Autodesk Fusion 360 part; units mm, degrees
sketch "Sketch1" plane through (0, 0, 0) normal (0, 0, 1) x (1, 0, 0)
  line L0 (-0.5032, -3.4999) -> (2.3969, -3.5062) construction
  line L1 (3.8936, -5.0095) -> (3.8707, -15.5094) construction
  line L2 (5.3674, -17.0127) -> (32.3673, -17.0717) construction
  line L3 (33.8706, -15.575) -> (33.8935, -5.075) construction
  line L4 (35.3968, -3.5783) -> (37.3968, -3.5826) construction
  line L5 (38.8935, -5.0859) -> (38.8706, -15.5859) construction
  line L6 (40.3673, -17.0892) -> (58.8673, -17.1296) construction
  arc A0 (3.8707, -15.5094) -> (5.3674, -17.0127) centre (5.3707, -15.5127) ccw construction
  arc A1 (3.8936, -5.0095) -> (2.3969, -3.5062) centre (2.3936, -5.0062) ccw construction
  arc A2 (32.3673, -17.0717) -> (33.8706, -15.575) centre (32.3706, -15.5717) ccw construction
  arc A3 (35.3968, -3.5783) -> (33.8935, -5.075) centre (35.3935, -5.0783) ccw construction
  arc A4 (38.8935, -5.0859) -> (37.3968, -3.5826) centre (37.3935, -5.0826) ccw construction
  arc A5 (38.8706, -15.5859) -> (40.3673, -17.0892) centre (40.3706, -15.5892) ccw construction
  arc A6 (4.6436, -5.0111) -> (2.3985, -2.7562) centre (2.3936, -5.0062) ccw
  line L7 (-0.5049, -4.2499) -> (2.3952, -4.2562)
  line L8 (-0.5016, -2.7499) -> (2.3985, -2.7562)
  arc A7 (3.1436, -5.0078) -> (2.3952, -4.2562) centre (2.3936, -5.0062) ccw
  line L9 (3.1436, -5.0078) -> (3.1207, -15.5078)
  arc A8 (3.1207, -15.5078) -> (5.3658, -17.7627) centre (5.3707, -15.5127) ccw
  line L10 (5.3658, -17.7627) -> (32.3657, -17.8217)
  line L11 (4.6436, -5.0111) -> (4.6207, -15.5111)
  arc A9 (4.6207, -15.5111) -> (5.369, -16.2627) centre (5.3707, -15.5127) ccw
  line L12 (5.369, -16.2627) -> (32.369, -16.3217)
  arc A10 (32.369, -16.3217) -> (33.1206, -15.5733) centre (32.3706, -15.5717) ccw
  line L13 (33.1206, -15.5733) -> (33.1435, -5.0734)
  arc A11 (35.3984, -2.8283) -> (33.1435, -5.0734) centre (35.3935, -5.0783) ccw
  line L14 (35.3984, -2.8283) -> (37.3984, -2.8326)
  arc A12 (39.6435, -5.0876) -> (37.3984, -2.8326) centre (37.3935, -5.0826) ccw
  line L15 (39.6435, -5.0876) -> (39.6206, -15.5875)
  arc A13 (39.6206, -15.5875) -> (40.3689, -16.3392) centre (40.3706, -15.5892) ccw
  line L16 (40.3689, -16.3392) -> (58.8689, -16.3796)
  arc A14 (32.3657, -17.8217) -> (34.6206, -15.5766) centre (32.3706, -15.5717) ccw
  line L17 (34.6206, -15.5766) -> (34.6435, -5.0766)
  arc A15 (35.3952, -4.3283) -> (34.6435, -5.0766) centre (35.3935, -5.0783) ccw
  line L18 (35.3952, -4.3283) -> (37.3952, -4.3326)
  arc A16 (38.1435, -5.0843) -> (37.3952, -4.3326) centre (37.3935, -5.0826) ccw
  line L19 (38.1435, -5.0843) -> (38.1206, -15.5843)
  arc A17 (38.1206, -15.5843) -> (40.3657, -17.8392) centre (40.3706, -15.5892) ccw
  line L20 (40.3657, -17.8392) -> (58.8656, -17.8796)
  line L21 (58.8689, -16.3796) -> (58.8656, -17.8796)
  line L22 (-0.5016, -2.7499) -> (-0.4994, -1.7499) construction
  line L23 (-0.5049, -4.2499) -> (-0.4939, 0.7501) construction
  arc A18 (-0.4972, -0.7499) -> (-0.5016, -2.7499) centre (-0.4994, -1.7499) ccw
  arc A19 (-0.4939, 0.7501) -> (-0.5049, -4.2499) centre (-0.4994, -1.7499) ccw
  line L24 (-0.4972, -0.7499) -> (1.5028, -0.7542)
  line L25 (-0.4939, 0.7501) -> (1.5061, 0.7458)
  arc A20 (1.5028, -0.7542) -> (1.5061, 0.7458) centre (1.5044, -0.0042) ccw
  point P0 (3.8969, -3.5095)
  point P1 (3.8674, -17.0094)
  point P2 (33.8673, -17.075)
  point P3 (33.8968, -3.575)
  point P4 (38.8968, -3.5859)
  point P5 (38.8673, -17.0859)
  dimension "d34" = 30
  dimension "d35" = 13.5
  dimension "d36" = 5
  dimension "d37" = 13.5
  dimension "d38" = 20
  dimension "d39" = 1.5
  dimension "d40" = 1.5
  dimension "d41" = 1.5
  dimension "d42" = 1.5
  dimension "d43" = 1.5
  dimension "d44" = 1.5
  dimension "d49" = 0.75
  dimension "d52" = 0.75
  dimension "d53" = -0.75
  dimension "d54" = -0.75
  dimension "d55" = 0.75
  dimension "d56" = -0.75
  dimension "d57" = 0.75
  dimension "d58" = 0.75
  dimension "d59" = 1
  dimension "d60" = 2
  dimension "d62" = 5
  dimension "d67" = 2
  dimension "d68" = 2
extrude "Extrude1" add sketch "Sketch1" along normal blind 20
mirror "Mirror1" about plane through (58.8689, -16.3796, 0) normal (1, -0.0022, 0) of bodies 1 merged
equation "i1 = 2 mm"
equation "i2 = 5 mm"
equation "i3 = 30 mm"
equation "d34 = i3"
equation "d35 = h - t"
equation "d36 = i2"
equation "d37 = h - t"
equation "d38 = i / 2 - 2 * i2 - i3"
equation "d39 = Radial Dimension-2"
equation "d40 = Radial Dimension-3"
equation "d41 = Radial Dimension-4"
equation "d42 = Radial Dimension-5"
equation "d43 = Radial Dimension-6"
equation "d44 = Radial Dimension-7"
equation "d49 = t / 2"
equation "d52 = t / 2"
equation "d53 = -t / 2"
equation "d54 = -t / 2"
equation "d55 = t / 2"
equation "d56 = -t / 2"
equation "d57 = t / 2"
equation "d58 = t / 2"
equation "d67 = i1"
equation "d68 = i1"
Read the model definition and answer for the solid it produces. Units are mm, in the model's axes. A direction names the side the tool comes from. Round coordinates to 2 decimals unless told otherwise and drop trailing zeros. Order: outer loops, then holes, each group sorted by start corner. A loop starts at its lowest first (then second) coordinate and runs counter-clockwise, first axis right, second up.
1) The part is cut by section B-B on x = 94.5. Write down the section's boundary in (y, z).
2) Flat-ended cylindrical pins translate along their axes: pin 1 (10 mm diameter, centred on x = 73.5, z = 3.5, fed in from +Y); pin 2 (5 mm diameter, centred on y = -10, z = 14.5, fed in from +X); pin 3 (6 mm diameter, centred on x = 20, z = 7.5, fed in from +Y). Find the tip coordinate at first contact, or state that the pin passes through.
3) Straight lines are drawn through the part: L1, parallel to X at y = -5.5, z = 10.5; L2, parallel to X at y = -5, z = 3; L3, parallel to Y at x = 91.5, z = 4.5. For each, find the intervals that lie inside material, in ascending order.
4) For faces 1 (the face through (33.976, -17.149, 9.86)), 2 (the face through (59, -17, 20)), 3 (the face through (78.79, -3.6, 9.86)), determine the directions among +Z, -Z, +X, -X, +Y, -Y from which every point of the face is accessible in a straight line to the end or side of a thin tool.
5) The part is cut by section A-A on y = -13.5. Write down the section's boundary in (x, z), plus the area to 3 significant figures.
Resolved:
1. outline: (-17.96, 0) - (-16.46, 0) - (-16.46, 20) - (-17.96, 20) - close
2. pin 1: stops at y = -3.96
2. pin 2: stops at x = 114.64
2. pin 3: stops at y = -16.29
3. L1: x = 3.14 to 4.64, 33.14 to 34.64, 38.14 to 39.64, 78.14 to 79.64, 83.14 to 84.64, 113.14 to 114.64
3. L2: x = 3.14 to 4.64, 33.14 to 34.65, 38.14 to 39.64, 78.15 to 79.67, 83.12 to 84.64, 113.16 to 114.69
3. L3: y = -17.95 to -16.45
4. face 1: +Z, -Z, -Y
4. face 2: +Z, +X, -X, +Y, -Y
4. face 3: +Z, -Z, +Y
5. outline: (3.13, 0) - (4.63, 0) - (4.63, 20) - (3.13, 20) - close; (33.13, 0) - (34.63, 0) - (34.63, 20) - (33.13, 20) - close; (38.13, 0) - (39.63, 0) - (39.63, 20) - (38.13, 20) - close; (78.13, 0) - (79.63, 0) - (79.63, 20) - (78.13, 20) - close; (83.13, 0) - (84.63, 0) - (84.63, 20) - (83.13, 20) - close; (113.13, 0) - (114.63, 0) - (114.63, 20) - (113.13, 20) - close
5. area: 180 mm2
